```python
from build123d import *

# Parameters (mm, degrees)
ESQUISSE1_R             = 1
BOSS_EXTRU_1_DEPTH      = 6
ESQUISSE2_R             = 10
ESQUISSE2_R_2           = 2
ESQUISSE2_R_3           = 1.4
ESQUISSE2_R_4           = 1.5
ESQUISSE2_W             = 8
ESQUISSE2_H             = 55
ESQUISSE2_W_2           = 44
ENL_V_MAT_EXTRU_1_DEPTH = 6
ESQUISSE3_W             = 6
ESQUISSE3_H             = 10
ESQUISSE3_W_2           = 10
ESQUISSE3_H_2           = 6
ESQUISSE3_W_3           = 15
ENL_V_MAT_EXTRU_2_DEPTH = 6
ESQUISSE4_R             = 1.5
ENL_V_MAT_EXTRU_3_DEPTH = 6
ESQUISSE5_W             = 10
ESQUISSE5_H             = 6
ESQUISSE5_W_2           = 20
ENL_V_MAT_EXTRU_4_DEPTH = 6
ESQUISSE6_R             = 1.65
ESQUISSE6_R_2           = 1.5
ESQUISSE6_R_3           = 2
ENL_V_MAT_EXTRU_5_DEPTH = 6


with BuildPart() as part:
    # Esquisse1 → Boss.-Extru.1 (new body)
    with BuildSketch(Plane.XY):
        Polygon((-165, 96.73), (165, 96.73), (165, -18.27), (123, -109.022410436), (-123, -109.022410436), (-165, -18.27), align=None)
        with Locations((-23.6, -89.522410436)):
            Circle(ESQUISSE1_R, mode=Mode.SUBTRACT)
        with Locations((-23.6, -73.522410436)):
            Circle(ESQUISSE1_R, mode=Mode.SUBTRACT)
        with Locations((-39.6, -89.522410436)):
            Circle(ESQUISSE1_R, mode=Mode.SUBTRACT)
        with Locations((-39.6, -73.522410436)):
            Circle(ESQUISSE1_R, mode=Mode.SUBTRACT)
    extrude(amount=BOSS_EXTRU_1_DEPTH)

    # Esquisse2 → Enlèv. mat.-Extru.1 (cut)
    with BuildSketch(Plane.XY.offset(6)):
        with Locations((140, 76.73)):
            Circle(ESQUISSE2_R)
        with Locations((108, -89.022410436)):
            Circle(ESQUISSE2_R)
        with Locations(Location((-140, 76.73, 0), (0, 0, 180))):
            Circle(ESQUISSE2_R)
        with Locations(Location((-108, -89.022410436, 0), (0, 0, 180))):
            Circle(ESQUISSE2_R)
        with Locations((161, -16.022410436)):
            Circle(ESQUISSE2_R_2)
        with Locations((119, -105.022410436)):
            Circle(ESQUISSE2_R_2)
        with Locations((161, 92.73)):
            Circle(ESQUISSE2_R_2)
        with Locations(Location((-161, 92.73, 0), (0, 0, 180))):
            Circle(ESQUISSE2_R_2)
        with Locations(Location((-161, -16.022410436, 0), (0, 0, 180))):
            Circle(ESQUISSE2_R_2)
        with Locations(Location((-119, -105.022410436, 0), (0, 0, 180))):
            Circle(ESQUISSE2_R_2)
        with Locations((125.27, 76.73)):
            Circle(ESQUISSE2_R_3)
        with Locations((110.27, 76.73)):
            Circle(ESQUISSE2_R_3)
        with Locations((114.7893454, -75.950391119)):
            Circle(ESQUISSE2_R_4)
        with Locations((121.703139086, -62.638762485)):
            Circle(ESQUISSE2_R_4)
        with Locations(Location((-110.27, 76.73, 0), (0, 0, 180))):
            Circle(ESQUISSE2_R_3)
        with Locations(Location((-125.27, 76.73, 0), (0, 0, 180))):
            Circle(ESQUISSE2_R_3)
        with Locations(Location((-121.703139086, -62.638762485, 0), (0, 0, 180))):
            Circle(ESQUISSE2_R_4)
        with Locations(Location((-114.7893454, -75.950391119, 0), (0, 0, 180))):
            Circle(ESQUISSE2_R_4)
        with Locations((-154, 28.477589564)):
            Rectangle(ESQUISSE2_W, ESQUISSE2_H)
        with Locations((-108, 28.477589564)):
            Rectangle(ESQUISSE2_W_2, ESQUISSE2_H)
        with Locations((108, 28.477589564)):
            Rectangle(ESQUISSE2_W_2, ESQUISSE2_H)
        with Locations((154, 28.477589564)):
            Rectangle(ESQUISSE2_W, ESQUISSE2_H)
    extrude(amount=-ENL_V_MAT_EXTRU_1_DEPTH, mode=Mode.SUBTRACT)

    # Esquisse3 → Enlèv. mat.-Extru.2 (cut)
    with BuildSketch(Plane(origin=(0, 0, 0), x_dir=(-1, 0, 0), z_dir=(0, 0, -1))):
        with Locations((162, 1.73)):
            Rectangle(ESQUISSE3_W, ESQUISSE3_H)
        with Locations((162, 73.852589564)):
            Rectangle(ESQUISSE3_W, ESQUISSE3_H)
        with Locations((24.5, -106.022410436)):
            Rectangle(ESQUISSE3_W_2, ESQUISSE3_H_2)
        with Locations((-24.5, -106.022410436)):
            Rectangle(ESQUISSE3_W_2, ESQUISSE3_H_2)
        with Locations((-162, 73.852589564)):
            Rectangle(ESQUISSE3_W, ESQUISSE3_H)
        with Locations((-162, 1.73)):
            Rectangle(ESQUISSE3_W, ESQUISSE3_H)
        with Locations((107.5, 93.73)):
            Rectangle(ESQUISSE3_W_3, ESQUISSE3_H_2)
        with Locations((-42.5, 93.73)):
            Rectangle(ESQUISSE3_W_3, ESQUISSE3_H_2)
        with Locations((42.5, 93.73)):
            Rectangle(ESQUISSE3_W_3, ESQUISSE3_H_2)
        with Locations((-107.5, 93.73)):
            Rectangle(ESQUISSE3_W_3, ESQUISSE3_H_2)
    extrude(amount=-ENL_V_MAT_EXTRU_2_DEPTH, mode=Mode.SUBTRACT)

    # Esquisse4 → Enlèv. mat.-Extru.3 (cut)
    with BuildSketch(Plane(origin=(0, 0, 0), x_dir=(-1, 0, 0), z_dir=(0, 0, -1))):
        with Locations((162, -6.27)):
            Circle(ESQUISSE4_R)
        with Locations((0, -106.022410436)):
            Circle(ESQUISSE4_R)
        with Locations((162, 62.852589564)):
            Circle(ESQUISSE4_R)
        with Locations((0, 93.73)):
            Circle(ESQUISSE4_R)
        with Locations(Location((-39.25, -106.022410436, 0), (0, 0, 180))):
            Circle(ESQUISSE4_R)
        with Locations(Location((-14.75, -106.022410436, 0), (0, 0, 180))):
            Circle(ESQUISSE4_R)
        with Locations((14.75, -106.022410436)):
            Circle(ESQUISSE4_R)
        with Locations((39.25, -106.022410436)):
            Circle(ESQUISSE4_R)
        with Locations((150, 93.73)):
            Circle(ESQUISSE4_R)
        with Locations((125, 93.73)):
            Circle(ESQUISSE4_R)
        with Locations((90, 93.73)):
            Circle(ESQUISSE4_R)
        with Locations(Location((-25, 93.73, 0), (0, 0, 180))):
            Circle(ESQUISSE4_R)
        with Locations((60, 93.73)):
            Circle(ESQUISSE4_R)
        with Locations((25, 93.73)):
            Circle(ESQUISSE4_R)
        with Locations(Location((-60, 93.73, 0), (0, 0, 180))):
            Circle(ESQUISSE4_R)
        with Locations(Location((-90, 93.73, 0), (0, 0, 180))):
            Circle(ESQUISSE4_R)
        with Locations(Location((-125, 93.73, 0), (0, 0, 180))):
            Circle(ESQUISSE4_R)
        with Locations(Location((-150, 93.73, 0), (0, 0, 180))):
            Circle(ESQUISSE4_R)
        with Locations(Location((-162, 62.852589564, 0), (0, 0, 180))):
            Circle(ESQUISSE4_R)
        with Locations(Location((-162, -6.27, 0), (0, 0, 180))):
            Circle(ESQUISSE4_R)
    extrude(amount=-ENL_V_MAT_EXTRU_3_DEPTH, mode=Mode.SUBTRACT)

    # Esquisse5 → Enlèv. mat.-Extru.4 (cut)
    with BuildSketch(Plane(origin=(0, 0, 0), x_dir=(-1, 0, 0), z_dir=(0, 0, -1))):
        with Locations((114, -35.022410436)):
            Rectangle(ESQUISSE5_W, ESQUISSE5_H)
        with Locations((24, -35.022410436)):
            Rectangle(ESQUISSE5_W_2, ESQUISSE5_H)
        with Locations((-24, -35.022410436)):
            Rectangle(ESQUISSE5_W_2, ESQUISSE5_H)
        with Locations((-114, -35.022410436)):
            Rectangle(ESQUISSE5_W, ESQUISSE5_H)
    extrude(amount=-ENL_V_MAT_EXTRU_4_DEPTH, mode=Mode.SUBTRACT)

    # Esquisse6 → Enlèv. mat.-Extru.5 (cut)
    with BuildSketch(Plane(origin=(0, 0, 0), x_dir=(-1, 0, 0), z_dir=(0, 0, -1))):
        with Locations((-140, 3.477589564)):
            Circle(ESQUISSE6_R)
        with Locations((-140, 53.477589564)):
            Circle(ESQUISSE6_R)
        with Locations(Location((140, 53.477589564, 0), (0, 0, 180))):
            Circle(ESQUISSE6_R)
        with Locations(Location((140, 3.477589564, 0), (0, 0, 180))):
            Circle(ESQUISSE6_R)
        with Locations(Location((-39, -35.022410436, 0), (0, 0, 180))):
            Circle(ESQUISSE6_R_2)
        with Locations((9, -35.022410436)):
            Circle(ESQUISSE6_R_2)
        with Locations((39, -35.022410436)):
            Circle(ESQUISSE6_R_2)
        with Locations(Location((-9, -35.022410436, 0), (0, 0, 180))):
            Circle(ESQUISSE6_R_2)
        with Locations((-78.5, 49.477589564)):
            Circle(ESQUISSE6_R_3)
        with Locations((-78.5, 7.477589564)):
            Circle(ESQUISSE6_R_3)
        with Locations((-60, 47.977589564)):
            Circle(ESQUISSE6_R_3)
        with Locations((-60, 8.977894939)):
            Circle(ESQUISSE6_R_3)
        with Locations((60, 8.977894939)):
            Circle(ESQUISSE6_R_3)
        with Locations((60, 47.977589564)):
            Circle(ESQUISSE6_R_3)
        with Locations((-50, 45.977589564)):
            Circle(ESQUISSE6_R_3)
        with Locations((50, 45.977589564)):
            Circle(ESQUISSE6_R_3)
        with Locations((50, 10.977589564)):
            Circle(ESQUISSE6_R_3)
        with Locations((-50, 10.977589564)):
            Circle(ESQUISSE6_R_3)
        with Locations(Location((78.5, 7.477589564, 0), (0, 0, 180))):
            Circle(ESQUISSE6_R_3)
        with Locations(Location((78.5, 49.477589564, 0), (0, 0, 180))):
            Circle(ESQUISSE6_R_3)
        with Locations((104.5, -27.222410436)):
            Circle(ESQUISSE6_R_2)
        with Locations((104.5, -50.222410436)):
            Circle(ESQUISSE6_R_2)
        with Locations(Location((-104.5, -50.222410436, 0), (0, 0, 180))):
            Circle(ESQUISSE6_R_2)
        with Locations(Location((-104.5, -27.222410436, 0), (0, 0, 180))):
            Circle(ESQUISSE6_R_2)
    extrude(amount=-ENL_V_MAT_EXTRU_5_DEPTH, mode=Mode.SUBTRACT)


solid = part.part
```
For this review, take the finished solid that the model builds, in its own axes (mm). A direction names the side the tool comes from. Round coordinates to 2 decimals unless told otherwise and drop trailing zeros. Write each loop counter-clockwise with the first axis right and the second up, starting at its lowest first coordinate (ties: lowest second). Pieces come first, ordered by that corner, then holes. Notation, with made-up numbers: (-32.75, -30.75) - (20.25, -30.75) arc R24 cw to (20.25, 4.25) - close; hole circle Ø2 at (44.25, 81.25). An arc over 180 degrees is marked (long way). Answer as CSV lines item,"result". Start each with the question number.
(1) Mouldability with a two-part tool opening along X and no side actions: class faces 5 (the flat face through (162, 78.853, 3)), 6 (the flat face through (144.3, -63, 3)), 7 (the flat face through (24, -38.022, 3)), 8 (the flat face through (-86, 28, 3)) as +X half, -X half, draft (parallel to the pull), parting line (faces both ways), or undercut.
(2) For line 1 (Y direction, x = -14.75, z = 4.2); line 2 (Y direction, x = 30, z = 2.4); line 3 (X direction, y = 43, z = 1), list the stretches that pass through material, from the lowest coordinate up.
(3) Add section B-B, the plane z = 1.1. State how many separate pieces and enclosed holes the cut face has, plus the area to 3 significant figures.
(4) Machinability: for faces 1 (the flat face through (-107, 90.73, 3)), 2 (the flat face through (-24, -103.022, 3)), 3 (the flat face through (150, 28, 3)), 4 (the flat face through (162, 6.73, 3)), which of the approach directions +Z, -Z, +X, -X, +Y, -Y give a long, thin tool a straight path to every point of the face, cutting with its end or side? Answer none if there is none.
(5) Add section A-A, the plane y = 24.5. State the section outline as (x, z) points.
(6) For pin 1 (3 mm diameter, centred on x = 24, z = 4, fed in from -Y); pin 2 (3.5 mm diameter, centred on x = 14.75, y = -106.02, fed in from -Z), all flat-tipped, find the tip position at first contact; note any pin that passes through.
From the geometry:
1,face 5,"draft"
1,face 6,"+X half"
1,face 7,"undercut"
1,face 8,"undercut"
2,line 1,"y = -109.02 to -107.52, -104.52 to -38.02, -32.02 to 96.73"
2,line 2,"y = -109.02 to -38.02, -32.02 to 96.73"
2,line 3,"x = -165 to -158, -150 to -130, -86 to 86, 130 to 150, 158 to 165"
3,separate pieces,"1"
3,enclosed holes,"74"
3,area,"55,500 mm²"
4,face 1,"+Z, -Z, +Y"
4,face 2,"+Z, -Z, -Y"
4,face 3,"+Z, -Z"
4,face 4,"+Z, -Z, +X"
5,outline,"(-165, 0) - (-158, 0) - (-158, 6) - (-165, 6) - close; (-150, 0) - (-130, 0) - (-130, 6) - (-150, 6) - close; (-86, 0) - (86, 0) - (86, 6) - (-86, 6) - close; (130, 0) - (150, 0) - (150, 6) - (130, 6) - close; (158, 0) - (165, 0) - (165, 6) - (158, 6) - close"
6,pin 1,"stops at y = -103.02"
6,pin 2,"stops at z = 0"
